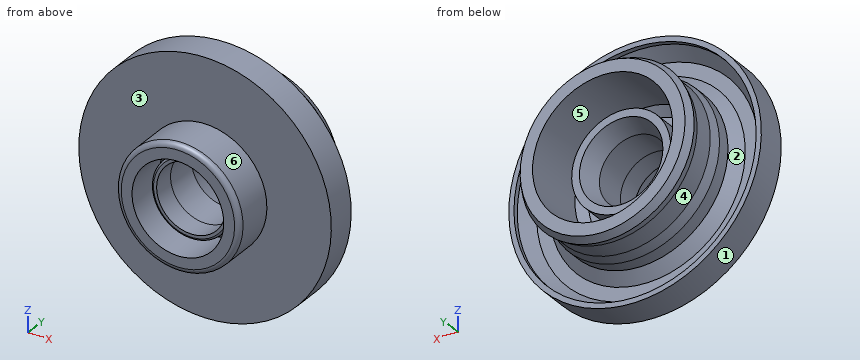
from build123d import *

# Parameters (mm, degrees)
SKETCH4_R           = 3.85
SKETCH4_R_2         = 3.35
BOSS_EXTRUDE1_DEPTH = 2.1
FILLET1_R           = 0.5
FILLET2_R           = 0.2


with BuildPart() as part:
    # Sketch1 → Revolve1 (revolve)
    with BuildSketch(Plane.XY, mode=Mode.PRIVATE) as revolve1_sk:
        Polygon((-12.25, 7.1), (-4.45, 7.1), (-4.45, 0), (-6, 0), (-6, 4.1), (-12.25, 4.1), align=None)
    revolve(revolve1_sk.sketch.rotate(Axis((0, 0, 0), (0, 1, 0)), 270), axis=Axis((0, 0, 0), (0, 1, 0)))

    # Sketch2 → Cut-Revolve1 (revolve, cut)
    with BuildSketch(Plane.XY, mode=Mode.PRIVATE) as cut_revolve1_sk:
        Polygon((-11.75, 7.1), (-11.75, 6.6), (-10.769709447, 5.2), (-6.8, 5.2), (-6.8, 4.8), (0, 4.8), (0, 10.778180343), (-11.75, 10.778180343), align=None)
    revolve(cut_revolve1_sk.sketch.rotate(Axis((0, 4.8, 0), (0, 1, 0)), 270), axis=Axis((0, 4.8, 0), (0, 1, 0)), mode=Mode.SUBTRACT)

    # Sketch3 → Revolve2 (revolve)
    with BuildSketch(Plane.XY, mode=Mode.PRIVATE) as revolve2_sk:
        Polygon((-4.8, 9.2), (-4.8, 4.1), (-3.35, 4.1), (-3.35, 7.276765806), (-4.05, 9.2), align=None)
    revolve(revolve2_sk.sketch.rotate(Axis((0, 0, 0), (0, 1, 0)), 270), axis=Axis((0, 0, 0), (0, 1, 0)))

    # Sketch4 → Boss-Extrude1 (add)
    with BuildSketch(Plane.XZ.offset(-4.1)):
        with Locations(Location((0, 0, 0), (0, 0, 90))):
            Circle(SKETCH4_R)
        with Locations(Location((0, 0, 0), (0, 0, 270))):
            Circle(SKETCH4_R_2, mode=Mode.SUBTRACT)
    extrude(amount=BOSS_EXTRUDE1_DEPTH)

    # Sketch5 → Revolve3 (revolve)
    with BuildSketch(Plane.XY, mode=Mode.PRIVATE) as revolve3_sk:
        Polygon((-8, 12), (-6.8, 12), (-6.8, 5.2), (-9.469709447, 5.2), (-8.45, 6.219709447), (-8.45, 7.5), (-8.2, 8.5), (-8.2, 10.5), (-8.4, 11.246410162), align=None)
    revolve(revolve3_sk.sketch.rotate(Axis((0, 0, 0), (0, 1, 0)), 270), axis=Axis((0, 0, 0), (0, 1, 0)))

    # Sketch6 → Revolve4 (revolve)
    with BuildSketch(Plane.XY, mode=Mode.PRIVATE) as revolve4_sk:
        Polygon((-6.8, 5.6), (-6, 4.8), (-6, 4.543753343), (-7.17505457, 4.543753343), (-7.17505457, 5.6), align=None)
    revolve(revolve4_sk.sketch.rotate(Axis((0, 0, 0), (0, 1, 0)), 270), axis=Axis((0, 0, 0), (0, 1, 0)))

    # Fillet1
    fillet1_edges = [part.edges().sort_by_distance(p)[0] for p in [
        (0, 0, 6),
    ]]
    fillet(fillet1_edges, radius=FILLET1_R)

    # Fillet2
    fillet2_edges = [part.edges().sort_by_distance(p)[0] for p in [
        (0, 2, -3.85),
    ]]
    fillet(fillet2_edges, radius=FILLET2_R)


solid = part.part
The model under review builds one solid part; all positions refer to its coordinate system, in mm. Face numbers are marked on the shaded views. A direction names the side the tool comes from. Coordinates: 2 decimals unless noted, no trailing zeros. Loops run counter-clockwise (first coordinate to the right, second up) from the corner with the lowest first, then second, coordinate; pieces in that order, holes last. Notation, with made-up numbers: M 32.25,1.25 L 69.25,1.25 A25 cw 69.25,21.25 Z; hole C 49,55 d11. An arc over 180 degrees is marked long. Put each result on its own line as item: value. Start each with the question number.
Q1. Clearance check with flat-ended pins moving along their axes: pin 1 (3 mm diameter, centred on x = -5, y = 7.5, fed in from -Z); pin 2 (5.5 mm diameter, centred on x = 0, z = 0, fed in from -Y); pin 3 (4 mm diameter, centred on x = -6.5, y = 2.5, fed in from -Z); pin 4 (5 mm diameter, centred on y = 5.5, z = -9.5, fed in from -X). State where each tip first meets the part, or that it passes through.
Q2. For the marked faces 4, 5 and 6, list the 3-axis set-ups (+Z, -Z, +X, -X, +Y, -Y) from which the entire face can be reached by the end or side of a thin tool; tool diameter is ignored.
Q3. Add section A-A (y = 1.5). Write out the cut boundary in (x, z), and give its area (3 significant figures).
Q4. Wall thickness on line 1 (X direction, y = 2.35, z = 0); line 2 (X direction, y = 6.25, z = 4); line 3 (Z direction, x = 3.75, y = 6): over which ranges is each line inside the solid? List them lowest first.
Q5. The part is to be moulded in two halves that separate along X. For the marked faces 1, 2 and 3, say which applies: +X half, -X half, draft (parallel to the pull), parting line (faces both ways), or undercut.
Answers:
1. pin 1: stops at z = -11.72
1. pin 2: passes through
1. pin 3: stops at z = -11.04
1. pin 4: stops at x = -10.05
2. face 4: none
2. face 5: +Y
2. face 6: -Y
3. outline: C 0,0 d12; hole C 0,0 d8.9
3. area: 50.9 mm^2
4. line 1: x = -6 to -4.45, -3.85 to -3.35, 3.35 to 3.85, 4.45 to 6
4. line 2: x = -11.58 to -10.79, -7.44 to -5.5, -2.65 to 2.65, 5.5 to 7.44, 10.79 to 11.58
4. line 3: z = -11.66 to -10.69, -7.82 to -5.67, -3 to 3, 5.67 to 7.82, 10.69 to 11.66
5. face 1: parting line
5. face 2: undercut
5. face 3: draft
